Source: CAD feature listing. Evaluate the final solid. Frame: model axes, mm. A direction names the side the tool comes from. Round coordinates to 2 decimals unless told otherwise and drop trailing zeros. Order: outer loops, then holes, each group sorted by start corner. A loop starts at its lowest first (then second) coordinate and runs counter-clockwise, first axis right, second up. Notation, with made-up numbers: (-32, -39.5) -> (-11, -39.5) arc R13 cw to (-11, -32.5) -> close; hole circle Ø8 at (9.25, 82.25). An arc over 180 degrees is marked (long way). Answer as CSV lines item,"result".
from build123d import *

# Parameters (mm, degrees)
BOSS_EXTRUDE1_DEPTH = 2
SKETCH2_R           = 5
BOSS_EXTRUDE3_DEPTH = 4
SKETCH5_R           = 3
CUT_EXTRUDE1_DEPTH  = 4
SKETCH6_R           = 1.5
CUT_EXTRUDE2_DEPTH  = 2
SKETCH8_R           = 2.5
CUT_EXTRUDE3_DEPTH  = 3
SKETCH7_R           = 2.5
CUT_EXTRUDE4_DEPTH  = 3


with BuildPart() as part:
    # Sketch1 → Boss-Extrude1 (new body)
    with BuildSketch(Plane(origin=(0, 0, 0), x_dir=(1, 0, 0), z_dir=(0, 1, 0))):
        with BuildLine():
            Line((-20, 7.598649923), (20, 7.598649923))
            ThreePointArc((20, 7.598649923), (27.5, 0.098649923), (20, -7.401350077))
            Line((20, -7.401350077), (-20, -7.401350077))
            ThreePointArc((-20, -7.401350077), (-27.5, 0.098649923), (-20, 7.598649923))
        make_face()
    extrude(amount=BOSS_EXTRUDE1_DEPTH)

    # Sketch2 → Boss-Extrude3 (add)
    with BuildSketch(Plane(origin=(0, 2, 0), x_dir=(1, 0, 0), z_dir=(0, 1, 0))):
        Circle(SKETCH2_R)
    extrude(amount=BOSS_EXTRUDE3_DEPTH)

    # Sketch5 → Cut-Extrude1 (cut)
    with BuildSketch(Plane(origin=(0, 6, 0), x_dir=(1, 0, 0), z_dir=(0, 1, 0))):
        Circle(SKETCH5_R)
    extrude(amount=-CUT_EXTRUDE1_DEPTH, mode=Mode.SUBTRACT)

    # Sketch6 → Cut-Extrude2 (cut)
    with BuildSketch(Plane(origin=(0, 2, 0), x_dir=(1, 0, 0), z_dir=(0, 1, 0))):
        Circle(SKETCH6_R)
    extrude(amount=-CUT_EXTRUDE2_DEPTH, mode=Mode.SUBTRACT)

    # Sketch8 → Cut-Extrude3 (cut, through all)
    with BuildSketch(Plane(origin=(0, 2, 0), x_dir=(1, 0, 0), z_dir=(0, 1, 0))):
        with Locations((-12.2, 0.009046723)):
            Circle(SKETCH8_R)
    extrude(amount=-CUT_EXTRUDE3_DEPTH, mode=Mode.SUBTRACT)

    # Sketch7 → Cut-Extrude4 (cut, through all)
    with BuildSketch(Plane(origin=(0, 2, 0), x_dir=(1, 0, 0), z_dir=(0, 1, 0))):
        with Locations((12.2, 0)):
            Circle(SKETCH7_R)
    extrude(amount=-CUT_EXTRUDE4_DEPTH, mode=Mode.SUBTRACT)


solid = part.part
1. Mould query, pull axis X, two halves, no side actions, for faces 3 (the cylindrical face through (-1.08, 3.97, 4.88)), 4 (the cylindrical face through (14.585, 1.014, -0.751)), 5 (the flat face through (0, 0, -2)), 6 (the cylindrical face through (-14.7, 1, -0.1)). Classes: released by +X, released by -X, zero draft, split by the parting line, or undercut.
Results below:
face 3,"split by the parting line"
face 4,"undercut"
face 5,"zero draft"
face 6,"undercut"
2. Section query B-B on y = 1.35. Return loops of the section in (x, z), and give its area (3 significant figures).
Results below:
outline,"(-20, -7.6) -> (20, -7.6) arc R7.5 ccw to (20, 7.4) -> (-20, 7.4) arc R7.5 ccw to start; hole circle Ø5 at (-12.2, -0.01); hole circle Ø3 at (0, 0); hole circle Ø5 at (12.2, 0)"
area,"730 mm2"
3. Line query: L1, parallel to X at y = 1.1, z = 0; L2, parallel to Z at x = 12.2, y = 0.65; L3, parallel to Z at x = 0, y = 0.9. Output: solid intervals per line, ascending. Write a range as [from, to].
Results below:
L1,"[-27.5, -14.7], [-9.7, -1.5], [1.5, 9.7], [14.7, 27.5]"
L2,"[-7.6, -2.5], [2.5, 7.4]"
L3,"[-7.6, -1.5], [1.5, 7.4]"
4. Section query A-A on x = 12.2. Return loops of the section in (y, z), and give its area (3 significant figures).
Results below:
outline,"(0, -7.6) -> (2, -7.6) -> (2, -2.5) -> (0, -2.5) -> close; (0, 2.5) -> (2, 2.5) -> (2, 7.4) -> (0, 7.4) -> close"
area,"20.0 mm2"
5. Pin query (flat end, axial travel): pin 1 (5 mm diameter, centred on x = 0, z = 0, fed in from +Y); pin 2 (2 mm diameter, centred on y = 2, z = 1.5, fed in from +X). Return the tip coordinate at first contact, or that it passes through.
Results below:
pin 1,"y = 2"
pin 2,"x = 27.48"
6. Section query D-D on x = 0. Return loops of the section in (y, z).
Results below:
outline,"(0, -7.6) -> (2, -7.6) -> (2, -5) -> (6, -5) -> (6, -3) -> (2, -3) -> (2, -1.5) -> (0, -1.5) -> close; (0, 1.5) -> (2, 1.5) -> (2, 3) -> (6, 3) -> (6, 5) -> (2, 5) -> (2, 7.4) -> (0, 7.4) -> close"
7. Reachability of faces 1 (the cylindrical face through (-3, 4, 0)), 2 (the flat face through (-0.1, 6, 3.3)) from +Z, -Z, +X, -X, +Y, -Y: full face, straight path, thin tool, end or side. Return the list, or none.
Results below:
face 1,"+Y"
face 2,"+Z, -Z, +X, -X, +Y"
8. Section query C-C on x = -8.5. Return loops of the section in (y, z).
Results below:
outline,"(0, -7.6) -> (2, -7.6) -> (2, 7.4) -> (0, 7.4) -> close"
